Can you work these out from the model? Positions are in its coordinate system, mm. A direction names the side the tool comes from. Give positions to 0.01 mm unless a question says otherwise; leave off trailing zeros. Write each loop counter-clockwise with the first axis right and the second up, starting at its lowest first coordinate (ties: lowest second). Pieces come first, ordered by that corner, then holes. Notation, with made-up numbers: (67.5, 30) - (115.5, 30) arc R16 cw to (115.5, 48) - close; hole circle Ø1 at (-23.5, 60). An arc over 180 degrees is marked (long way). Use a Markdown table: item, result. Add a question column.
```python
from build123d import *
from build123d import SkipClean  # not in build123d's __all__

# Parameters (mm, degrees)
F1_DEPTH       = 2
F2_DEPTH       = 25
F3_T1_DEPTH    = 29
F3_T3_DEPTH    = 29
F3_T5_DEPTH    = 29
F3_T7_DEPTH    = 29
F3_T9_DEPTH    = 43.2
F3_T11_DEPTH   = 43.2
F3_T13_DEPTH   = 50
F4_R           = 2
F5_SIZE        = 2
F7_D           = 3.3
F7_CSINK_D     = 6
F7_CSINK_ANGLE = 90


# Not quite as in the source:
# - a fillet or chamfer that OpenCascade refuses, or shapes differently, is made with other operations: its cross-section is extruded or revolved along the edge and cut away or added
# - a feature names something its author has since deleted; it is built from what else it names


with BuildPart() as f1:
    # F0 (on Top) → F1 (new body)
    with BuildSketch(Plane.XY):
        Polygon((5.1, 0), (5.1, 10.2), (5.1, 32.5735770881), (-5.1, 32.5735770881), (-5.1, 10.2), (-27.6520505063, 10.2), (-27.6520505063, 0), (0, 0), align=None)
        Polygon((5.1, 32.5735770881), (5.1, 10.2), (5.1, 0), (0, 0), (-27.6520505063, 0), (-27.6520505063, -4), (0, -4), (9.1, -4), (9.1, 32.5735770881), align=None)
        Polygon((-5.1, 10.2), (-5.1, 32.5735770881), (-9.1, 32.5735770881), (-9.1, 14.2), (-27.6520505063, 14.2), (-27.6520505063, 10.2), align=None)
    extrude(amount=F1_DEPTH)

    # F0 (on Top) → F2 (join)
    with BuildSketch(Plane.XY):
        Polygon((-5.1, 10.2), (-5.1, 32.5735770881), (-9.1, 32.5735770881), (-9.1, 14.2), (-27.6520505063, 14.2), (-27.6520505063, 10.2), align=None)
        Polygon((5.1, 32.5735770881), (5.1, 10.2), (5.1, 0), (0, 0), (-27.6520505063, 0), (-27.6520505063, -4), (0, -4), (9.1, -4), (9.1, 32.5735770881), align=None)
    extrude(amount=F2_DEPTH)

    # F3: fillet of radius 5 on 7 edges, made by hand

    # F3_s2 → F3_t1 (cut)
    with BuildSketch(Plane.XZ.offset(-12.5)):
        with BuildLine():
            ThreePointArc((-22.6520505063, 25), (-26.1875844123, 23.5355339059), (-27.6520505063, 20))
            Line((-27.6520505063, 20), (-27.6520505063, 25))
            Line((-27.6520505063, 25), (-22.6520505063, 25))
        make_face()
    extrude(amount=F3_T1_DEPTH, mode=Mode.SUBTRACT)

    # F3_s4 → F3_t3 (cut)
    with BuildSketch(Plane.XZ.offset(-26.7)):
        with BuildLine():
            ThreePointArc((-22.6520505063, 25), (-26.1875844123, 23.5355339059), (-27.6520505063, 20))
            Line((-27.6520505063, 20), (-27.6520505063, 25))
            Line((-27.6520505063, 25), (-22.6520505063, 25))
        make_face()
    extrude(amount=F3_T3_DEPTH, mode=Mode.SUBTRACT)

    # F3_s6 → F3_t5 (cut)
    with BuildSketch(Plane.YZ.offset(-21.6)):
        with BuildLine():
            ThreePointArc((27.5735770881, 25), (31.1091109941, 23.5355339059), (32.5735770881, 20))
            Line((32.5735770881, 20), (32.5735770881, 25))
            Line((32.5735770881, 25), (27.5735770881, 25))
        make_face()
    extrude(amount=F3_T5_DEPTH, mode=Mode.SUBTRACT)

    # F3_s8 → F3_t7 (cut)
    with BuildSketch(Plane.YZ.offset(-7.4)):
        with BuildLine():
            ThreePointArc((32.5735770881, 20), (31.1091109941, 23.5355339059), (27.5735770881, 25))
            Line((27.5735770881, 25), (32.5735770881, 25))
            Line((32.5735770881, 25), (32.5735770881, 20))
        make_face()
    with SkipClean():  # cleaning this boolean's faces spoils the solid; the shape is the same uncleaned
        extrude(amount=F3_T7_DEPTH, mode=Mode.SUBTRACT)

    # F3_s10 → F3_t9 (cut)
    with BuildSketch(Plane.XZ.offset(-26.7)):
        with BuildLine():
            ThreePointArc((-22.6520505063, 0), (-26.1875844123, 1.4644660941), (-27.6520505063, 5))
            Line((-27.6520505063, 5), (-27.6520505063, 0))
            Line((-27.6520505063, 0), (-22.6520505063, 0))
        make_face()
    extrude(amount=F3_T9_DEPTH, mode=Mode.SUBTRACT)

    # F3_s12 → F3_t11 (cut)
    with BuildSketch(Plane.YZ.offset(-21.6)):
        with BuildLine():
            ThreePointArc((27.5735770881, 0), (31.1091109941, 1.4644660941), (32.5735770881, 5))
            Line((32.5735770881, 5), (32.5735770881, 0))
            Line((32.5735770881, 0), (27.5735770881, 0))
        make_face()
    extrude(amount=F3_T11_DEPTH, mode=Mode.SUBTRACT)

    # F3_s14 → F3_t13 (cut)
    with BuildSketch(Plane.XY.offset(-12.5)):
        with BuildLine():
            ThreePointArc((4.1, -4), (7.6355339059, -2.5355339059), (9.1, 1))
            Line((9.1, 1), (9.1, -4))
            Line((9.1, -4), (4.1, -4))
        make_face()
    extrude(amount=F3_T13_DEPTH, mode=Mode.SUBTRACT)

    # F4
    f4_edges = [f1.edges().sort_by_distance(p)[0] for p in [
        (-9.1, 14.2, 12.5),
    ]]
    fillet(f4_edges, radius=F4_R)

    # F5
    f5_edges = [f1.edges().sort_by_distance(p)[0] for p in [
        (-5.1, 10.2, 13.5),
    ]]
    chamfer(f5_edges, length=F5_SIZE)

    # F7 (through all)
    with Locations(Plane(origin=(0, 0, 0), x_dir=(1, 0, 0), z_dir=(0, 0, -1))):
        with Locations((-15, -5.1), (0, -20.1)):
            CounterSinkHole(F7_D / 2, F7_CSINK_D / 2, counter_sink_angle=F7_CSINK_ANGLE)


solid = f1.part
```
Q1. Suppose I cut it at D-D (y = 25.5). Please give me the cut outline in (x, z).
Q2. If we mould it in two halves opening along X, with no side actions, what happens to faces 5 (the cylindrical face through (-7.128, 31.07, 23.574)), 6 (the flat face through (-5.1, 22, 13)), 7 (the flat face through (-27.652, 12, 12))? For each: released by +X, released by -X, zero draft, split by the parting line, or undercut.
Q3. Suppose I cut it at B-B (y = 5.1). Please give me the cut outline in (x, z), and give its area (3 significant figures).
Q4. Suppose I cut it at C-C (z = 3.75). Please give me the cut outline in (x, y).
Q5. If I drill on probe 1 along Y at (x, z) = (-13.5, 13.5); probe 2 along Y at (x, z) = (-15, 1.6); probe 3 along X at (y, z) = (20.1, 1.95), over which ranges is the centre line in solid material (lowest first)? Write a range as [from, to].
Q6. I'm going to push flat-ended pins straight in: P1, Ø16, axis at x = -10, y = 23, coming from the +Z side; P2, Ø4.5, axis at x = 0, y = 20.1, coming from the -Z side; P3, Ø5, axis at y = 25, z = 7, coming from the -X side; P4, Ø5.5, axis at x = -15, y = 5.1, coming from the -Z side. Where does each tip first touch, or does it pass through?
Q7. On a 3-axis mill with a long thin cutter (end or side, diameter ignored), from which of +Z, -Z, +X, -X, +Y, -Y can I reach the whole of each face in a straight line? I mean faces 1 (the flat face through (-19, 14.2, 12)), 2 (the flat face through (-7, 9, 2)), 3 (the flat face through (5.1, 17, 13)), 4 (the flat face through (-11, 0, 13)). Say none if no direction works.
Q8. Suppose I cut it at A-A (x = -15). Please give me the cut outline in (y, z), and give its area (3 significant figures).
Derived:
| question | item | result |
|---|---|---|
| 1 | outline | (-9.1, 0) - (9.1, 0) - (9.1, 25) - (5.1, 25) - (5.1, 2) - (-5.1, 2) - (-5.1, 25) - (-9.1, 25) - close |
| 2 | face 5 | zero draft |
| 2 | face 6 | undercut |
| 2 | face 7 | released by -X |
| 3 | outline | (-26.65, 2) arc R5 ccw to (-22.65, 0) - (-18, 0) - (-16.65, 1.35) - (-16.65, 2) - close; (-13.35, 1.35) - (-12, 0) - (9.1, 0) - (9.1, 25) - (5.1, 25) - (5.1, 2) - (-13.35, 2) - close |
| 3 | area | 153 mm² |
| 4 | outline | (-27.49, -4) - (4.1, -4) arc R5 ccw to (9.1, 1) - (9.1, 32.41) - (5.1, 32.41) - (5.1, 0) - (-27.49, 0) - close; (-27.49, 10.2) - (-7.1, 10.2) - (-5.1, 12.2) - (-5.1, 32.41) - (-9.1, 32.41) - (-9.1, 16.2) arc R2 cw to (-11.1, 14.2) - (-27.49, 14.2) - close |
| 5 | probe 1 | [-4, 0], [10.2, 14.2] |
| 5 | probe 2 | [-4, 3.45], [6.75, 14.2] |
| 5 | probe 3 | [-9.1, -1.65], [1.65, 9.1] |
| 6 | P1 | z = 25 |
| 6 | P2 | z = 0.75 |
| 6 | P3 | x = -9.1 |
| 6 | P4 | z = 0.25 |
| 7 | face 1 | +Z, -Z, -X, +Y |
| 7 | face 2 | +Z |
| 7 | face 3 | +Z, +Y |
| 7 | face 4 | +Z, -X |
| 8 | outline | (-4, 0) - (2.1, 0) - (3.45, 1.35) - (3.45, 2) - (0, 2) - (0, 25) - (-4, 25) - close; (6.75, 1.35) - (8.1, 0) - (14.2, 0) - (14.2, 25) - (10.2, 25) - (10.2, 2) - (6.75, 2) - close |
| 8 | area | 212 mm² |
